Here's the drawing with two shaded views (mm, measured from the low corner). I have some questions. A direction names the side the tool comes from. Round coordinates to 2 decimals unless told otherwise and drop trailing zeros. Order: outer loops, then holes, each group sorted by start corner. A loop starts at its lowest first (then second) coordinate and runs counter-clockwise, first axis right, second up.
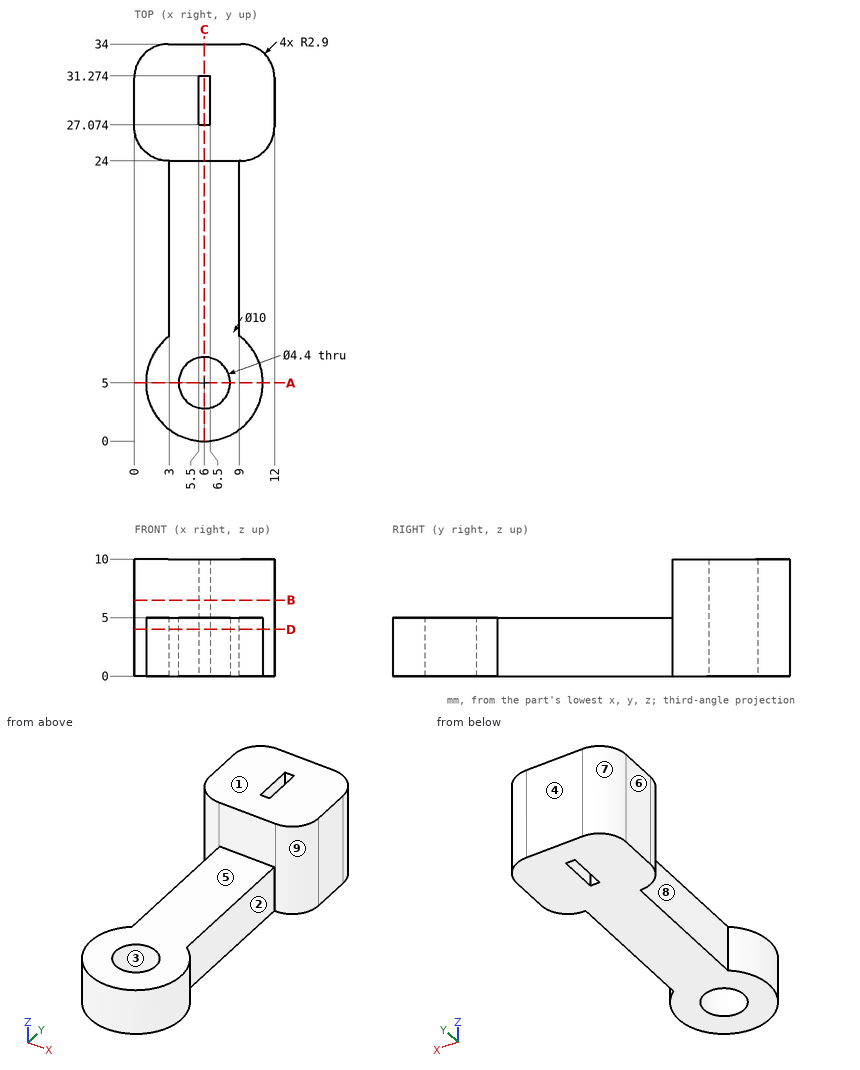
1. I'm going to push flat-ended pins straight in: P1, Ø1.5, axis at y = 7.5, z = 7, coming from the -X side; P2, Ø7, axis at x = 6, y = 5, coming from the +Z side; P3, Ø4, axis at y = 8, z = 5, coming from the +X side; P4, Ø4, axis at y = 15.5, z = 3.5, coming from the +X side. Where does each tip first touch, or does it pass through?
Evaluation:
P1: passes through
P2: stops at z = 5
P3: stops at x = 10.9
P4: stops at x = 9
2. If we section it at C-C, the plane x = 6: Write out the boundary of the cut face in (y, z), and give its area (3 significant figures).
Evaluation:
outline: (0, 0) - (2.8, 0) - (2.8, 5) - (0, 5) - close; (7.2, 0) - (27.07, 0) - (27.07, 10) - (24, 10) - (24, 5) - (7.2, 5) - close; (31.27, 0) - (34, 0) - (34, 10) - (31.27, 10) - close
area: 156 mm2
3. On a 3-axis mill with a long thin cutter (end or side, diameter ignored), from which of +Z, -Z, +X, -X, +Y, -Y can I reach the whole of each face in a straight line? I mean the marked faces 5, 6, 7, 8 and 9. Say none if no direction works.
Evaluation:
face 5: +Z, +X, -X, -Y
face 6: +Z, -Z, -X, +Y, -Y
face 7: +Z, -Z, -X, +Y
face 8: +Z, -Z, -X
face 9: +Z, -Z, +X
4. If we section it at D-D, the plane z = 4: Write out the boundary of the cut face in (x, y), and give its area (3 significant figures).
Evaluation:
outline: (0, 26.9) arc R2.9 ccw to (2.9, 24) - (3, 24) - (3, 9) arc R5 ccw (long way) to (9, 9) - (9, 24) - (9.1, 24) arc R2.9 ccw to (12, 26.9) - (12, 31.1) arc R2.9 ccw to (9.1, 34) - (2.9, 34) arc R2.9 ccw to (0, 31.1) - close; hole circle Ø4.4 at (6, 5); hole (5.5, 27.07) - (6.5, 27.07) - (6.5, 31.27) - (5.5, 31.27) - close
area: 258 mm2
5. I need wall thicknesses on probe 1 along Y at (x, z) = (6, 1.45); probe 2 along Z at (x, y) = (2.75, 8.5); probe 3 along Y at (x, z) = (3.5, 6). Which ranges of each line are inside material? Lowest first, please.
Evaluation:
probe 1: y = 0 to 2.8, 7.2 to 27.07, 31.27 to 34
probe 2: z = 0 to 5
probe 3: y = 24 to 34
6. If we section it at B-B, the plane z = 6.5: Write out the boundary of the cut face in (x, y).
Evaluation:
outline: (0, 26.9) arc R2.9 ccw to (2.9, 24) - (9.1, 24) arc R2.9 ccw to (12, 26.9) - (12, 31.1) arc R2.9 ccw to (9.1, 34) - (2.9, 34) arc R2.9 ccw to (0, 31.1) - close; hole (5.5, 27.07) - (6.5, 27.07) - (6.5, 31.27) - (5.5, 31.27) - close
7. If we section it at A-A, the plane y = 5: Write out the boundary of the cut face in (x, z), and give its area (3 significant figures).
Evaluation:
outline: (1, 0) - (3.8, 0) - (3.8, 5) - (1, 5) - close; (8.2, 0) - (11, 0) - (11, 5) - (8.2, 5) - close
area: 28.0 mm2
8. If we mould it in two halves opening along Y, with no side actions, what happens to the marked faces 1, 2, 3 and 4? For each: released by +Y, released by -Y, zero draft, split by the parting line, or undercut.
Evaluation:
face 1: zero draft
face 2: undercut
face 3: undercut
face 4: released by +Y
